Job drawing, mm, ordinate dimensions from the low corner. One solid piece. Give positions to 0.01 mm unless a question says otherwise; leave off trailing zeros. Loops run counter-clockwise (first coordinate to the right, second up) from the corner with the lowest first, then second, coordinate; pieces in that order, holes last. Notation, with made-up numbers: M 25,-30 L 30,-30 A21 ccw 30,-3 Z; hole C 2.25,81.5 d1. An arc over 180 degrees is marked long. Answer in a Markdown table with one row per item.
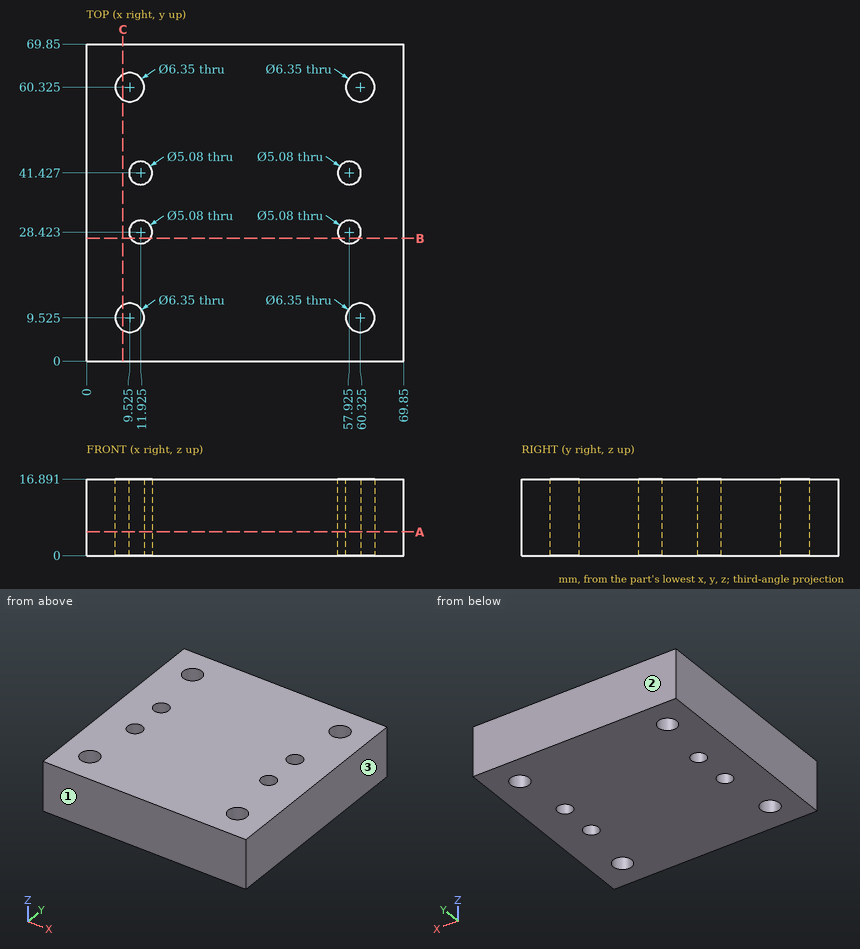
(1) Saw through at C-C (x = 8). Write the cut outline in (y, z), plus the area to 3 significant figures.
Recorded:
| item | result |
|---|---|
| outline | M 0,0 L 6.74,0 L 6.74,16.89 L 0,16.89 Z; M 12.31,0 L 57.54,0 L 57.54,16.89 L 12.31,16.89 Z; M 63.11,0 L 69.85,0 L 69.85,16.89 L 63.11,16.89 Z |
| area | 992 mm^2 |
(2) Saw through at B-B (y = 27). Write the cut outline in (x, z), plus the area to 3 significant figures.
Recorded:
| item | result |
|---|---|
| outline | M 0,0 L 9.82,0 L 9.82,16.89 L 0,16.89 Z; M 14.03,0 L 55.82,0 L 55.82,16.89 L 14.03,16.89 Z; M 60.03,0 L 69.85,0 L 69.85,16.89 L 60.03,16.89 Z |
| area | 1,040 mm^2 |
(3) Pull direction Y, two halves, no side cores. Call the marked faces 1, 2 and 3: +Y half, -Y half, draft (parallel to the pull), parting line (faces both ways), or undercut.
Recorded:
| item | result |
|---|---|
| face 1 | -Y half |
| face 2 | +Y half |
| face 3 | draft |
(4) Saw through at A-A (z = 5.25). Give the number of separate pieces and of enclosed holes in the cut face, plus the area to 3 significant figures.
Recorded:
| item | result |
|---|---|
| separate pieces | 1 |
| enclosed holes | 8 |
| area | 4,670 mm^2 |
(5) Drill centre lines: line 1 along Y through (x, z) = (62, 15); line 2 along X through (y, z) = (27.5, 2.5); line 3 along X through (y, z) = (42, 13.5). Where is each one in solid material? Low to high.
Recorded:
| item | result |
|---|---|
| line 1 | y = 0 to 6.83, 12.22 to 57.63, 63.02 to 69.85 |
| line 2 | x = 0 to 9.56, 14.29 to 55.56, 60.29 to 69.85 |
| line 3 | x = 0 to 9.45, 14.4 to 55.45, 60.4 to 69.85 |
